The listing builds one solid part. Answer for the finished solid, in the listing's coordinates (mm). A direction names the side the tool comes from. Coordinates: 2 decimals unless noted, no trailing zeros. Loops run counter-clockwise (first coordinate to the right, second up) from the corner with the lowest first, then second, coordinate; pieces in that order, holes last. Notation, with made-up numbers: (-32, -4) - (-9, -4) arc R12 cw to (-9, 5) - close; hole circle Ø3 at (82.25, 80.5). An arc over 180 degrees is marked (long way). Return JSON: item names as keys, results as strings. Group by question number.
1. The mould has two halves that part along X. Classify faces 1 (the face through (-0.05, -0.21, 5.28)), 2 (the face through (0, -2, 8)), 3 (the face through (0, 0, 0)): pulls with the +X half, pulls with the -X half, needs draft (parallel to the pull), parting line crosses it, or undercut.
2. Which of the six approach directions +Z, -Z, +X, -X, +Y, -Y give full straight-line access (tool end or side, diameter ignored) to faces 4 (the face through (-1.73, -7.81, 1.23)), 5 (the face through (-2, 4, 2.5))?
3. Each of these flat-tipped pins is pushed along its axis until it touches: P1, Ø1.5, axis at y = 1, z = 2.5, coming from the -X side; P2, Ø8, axis at x = -5, z = 11.5, coming from the +Y side; P3, Ø6, axis at y = -5.5, z = 8, coming from the -X side; P4, Ø4, axis at y = 2.5, z = 9.5, coming from the -X side. Where does it stop, or does it pass through?
4. Find the intervals of material crossed by line 1 along Y through (x, z) = (0, 1.05); line 2 along Y through (x, z) = (0, 9.75); line 3 along Z through (x, y) = (2.5, 1), in increasing order.
5. Section A-A (z = 7) is taken. Write down the section's boundary in (x, y), and give its area (3 significant figures).
```python
from build123d import *

# Parameters (mm, degrees)
SKETCH1_R                 = 8
BOSS_EXTRUDE1_DEPTH       = 2.5
SKETCH3_R                 = 4
BOSS_EXTRUDE2_DEPTH       = 0.3
SKETCH4_R                 = 2
BOSS_EXTRUDE3_DEPTH       = 11.6
M3X0_5_TAPPED_HOLE1_D     = 2.5
M3X0_5_TAPPED_HOLE1_DEPTH = 8.5
M3X0_5_TAPPED_HOLE1_TIP   = 0.751075774
SKETCH7_R                 = 1.5
CUT_EXTRUDE1_DEPTH        = 12.9
CUT_EXTRUDE1_DEPTH_BACK   = 3.5
FILLET1_R                 = 0.1


with BuildPart() as part:
    # Sketch1 → Boss-Extrude1 (new body)
    with BuildSketch(Plane.XY):
        Circle(SKETCH1_R)
    extrude(amount=BOSS_EXTRUDE1_DEPTH)

    # Sketch3 → Boss-Extrude2 (add)
    with BuildSketch(Plane.XY.offset(2.5)):
        Circle(SKETCH3_R)
    extrude(amount=BOSS_EXTRUDE2_DEPTH)

    # Sketch4 → Boss-Extrude3 (add)
    with BuildSketch(Plane.XY.offset(2.8)):
        Circle(SKETCH4_R)
    extrude(amount=BOSS_EXTRUDE3_DEPTH)

    # M3x0.5 Tapped Hole1
    with Locations(Plane.XY.offset(14.4)):
        with Locations((0, 0)):
            Hole(M3X0_5_TAPPED_HOLE1_D / 2, depth=M3X0_5_TAPPED_HOLE1_DEPTH)
            with Locations((0, 0, -(M3X0_5_TAPPED_HOLE1_DEPTH + M3X0_5_TAPPED_HOLE1_TIP / 2))):  # 118° drill point
                Cone(0, M3X0_5_TAPPED_HOLE1_D / 2, M3X0_5_TAPPED_HOLE1_TIP, mode=Mode.SUBTRACT)

    # Sketch7 → Cut-Extrude1 (cut, two sides)
    with BuildSketch(Plane.XY.offset(2.5)) as cut_extrude1_sk:
        with Locations((0, -6)):
            Circle(SKETCH7_R)
    extrude(amount=CUT_EXTRUDE1_DEPTH, mode=Mode.SUBTRACT)
    extrude(cut_extrude1_sk.sketch, amount=-CUT_EXTRUDE1_DEPTH_BACK, mode=Mode.SUBTRACT)

    # Fillet1
    fillet1_edges = [part.edges().sort_by_distance(p)[0] for p in [
        (-2, 0, 14.4),
        (-8, 0, 0),
        (-1.5, -6, 2.5),
        (-1.5, -6, 0),
        (-8, 0, 2.5),
    ]]
    fillet(fillet1_edges, radius=FILLET1_R)


solid = part.part
```
The answers:
{
 "1": {"face 1": "undercut", "face 2": "parting line crosses it", "face 3": "needs draft"},
 "2": {"face 4": "+Z, -Z", "face 5": "+Z"},
 "3": {"P1": "stops at x = -8", "P2": "stops at y = 1.73", "P3": "passes through", "P4": "stops at x = -1.94"},
 "4": {"line 1": "y = -8 to -7.5, -4.5 to 8", "line 2": "y = -2 to -1.25, 1.25 to 2", "line 3": "z = 0 to 2.8"},
 "5": {"outline": "circle Ø4 at (0, 0); hole circle Ø2.5 at (0, 0)", "area": "7.66 mm2"}
}
